from build123d import *


with BuildPart() as part:
    # Эскиз2 → Повернуть1 (revolve)
    with BuildSketch(Plane(origin=(0, 0, 0), x_dir=(0, 0, -1), z_dir=(1, 0, 0))):
        with BuildLine():
            Line((7.7, -7.5), (7.7, -6.5))
            Line((7.7, -6.5), (8.7, -6.5))
            Line((8.7, -6.5), (8.7, -7.5))
            Line((8.7, -7.5), (11.5, -7.5))
            ThreePointArc((11.5, -7.5), (11.853553391, -7.353553391), (12, -7))
            Line((12, -7), (12, -4))
            Line((12, -4), (-12, -4))
            Line((-12, -4), (-12, -7))
            ThreePointArc((-12, -7), (-11.853553391, -7.353553391), (-11.5, -7.5))
            Line((-11.5, -7.5), (-8.7, -7.5))
            Line((-8.7, -7.5), (-8.7, -6.5))
            Line((-8.7, -6.5), (-7.7, -6.5))
            Line((-7.7, -6.5), (-7.7, -7.5))
            Line((-7.7, -7.5), (7.7, -7.5))
        make_face()
    revolve(axis=Axis((0, 0, 12), (0, 0, -1)))


solid = part.part
Design review of the part built by this model. Coordinates are the model's own, in mm. A direction names the side the tool comes from. Coordinates: 2 decimals unless noted, no trailing zeros. Order: outer loops, then holes, each group sorted by start corner. A loop starts at its lowest first (then second) coordinate and runs counter-clockwise, first axis right, second up. Notation, with made-up numbers: (45, 63.5) - (63, 63.5) arc R20 ccw to (63, 68.5) - close; hole circle Ø1 at (7, 71). An arc over 180 degrees is marked (long way). Put each result on its own line as item: value.
1) Insertion check: P1, Ø5, axis at y = 5.5, z = 7.5, coming from the -X side; P2, Ø5, axis at y = -4.5, z = 1.5, coming from the -X side; P3, Ø5, axis at x = -6, z = 3.5, coming from the -Y side. Each pin has a flat end and moves straight along its axis. Give the tip position at first contact, or say it passes through.
Response values:
P1: stops at x = -6.87
P2: stops at x = -7.23
P3: stops at y = -6.63
2) Wall thickness on L1, parallel to Z at x = 2.5, y = -6.25; L2, parallel to X at y = 0, z = 5.5: over which ranges is each line inside the solid? List them lowest first. Write a range as from..to.
Response values:
L1: z = -12..-8.7, -7.7..7.7, 8.7..12
L2: x = -7.5..-4, 4..7.5
3) Take a section at C-C, the plane z = 1.25. Give the boundary of the cut face in (x, y).
Response values:
outline: circle Ø15 at (0, 0); hole circle Ø8 at (0, 0)
4) Take a section at D-D, the plane z = -8. Give the boundary of the cut face in (x, y).
Response values:
outline: circle Ø13 at (0, 0); hole circle Ø8 at (0, 0)
5) The part is to be moulded in two halves that separate along Z. For faces 3 (the face through (3.955, 5.158, 8.193)), 4 (the face through (-0.33, 7.493, 10.08)), 5 (the face through (3, -3, -12)), say which applies: released by +Z, released by -Z, zero draft, split by the parting line, or undercut.
Response values:
face 3: undercut
face 4: zero draft
face 5: released by -Z
6) Take a section at A-A, the plane y = 0. Give the boundary of the cut face in (x, z).
Response values:
outline: (-7.5, -11.5) arc R0.5 ccw to (-7, -12) - (-4, -12) - (-4, 12) - (-7, 12) arc R0.5 ccw to (-7.5, 11.5) - (-7.5, 8.7) - (-6.5, 8.7) - (-6.5, 7.7) - (-7.5, 7.7) - (-7.5, -7.7) - (-6.5, -7.7) - (-6.5, -8.7) - (-7.5, -8.7) - close; (4, -12) - (7, -12) arc R0.5 ccw to (7.5, -11.5) - (7.5, -8.7) - (6.5, -8.7) - (6.5, -7.7) - (7.5, -7.7) - (7.5, 7.7) - (6.5, 7.7) - (6.5, 8.7) - (7.5, 8.7) - (7.5, 11.5) arc R0.5 ccw to (7, 12) - (4, 12) - close
7) Tool access review of faces 1 (the face through (-3, 6, -7.7)), 2 (the face through (3.905, 0.867, 0.168)): name each direction out of +Z, -Z, +X, -X, +Y, -Y from which nothing blocks a thin tool from reaching the whole face with its end or side.
Response values:
face 1: none
face 2: +Z, -Z
